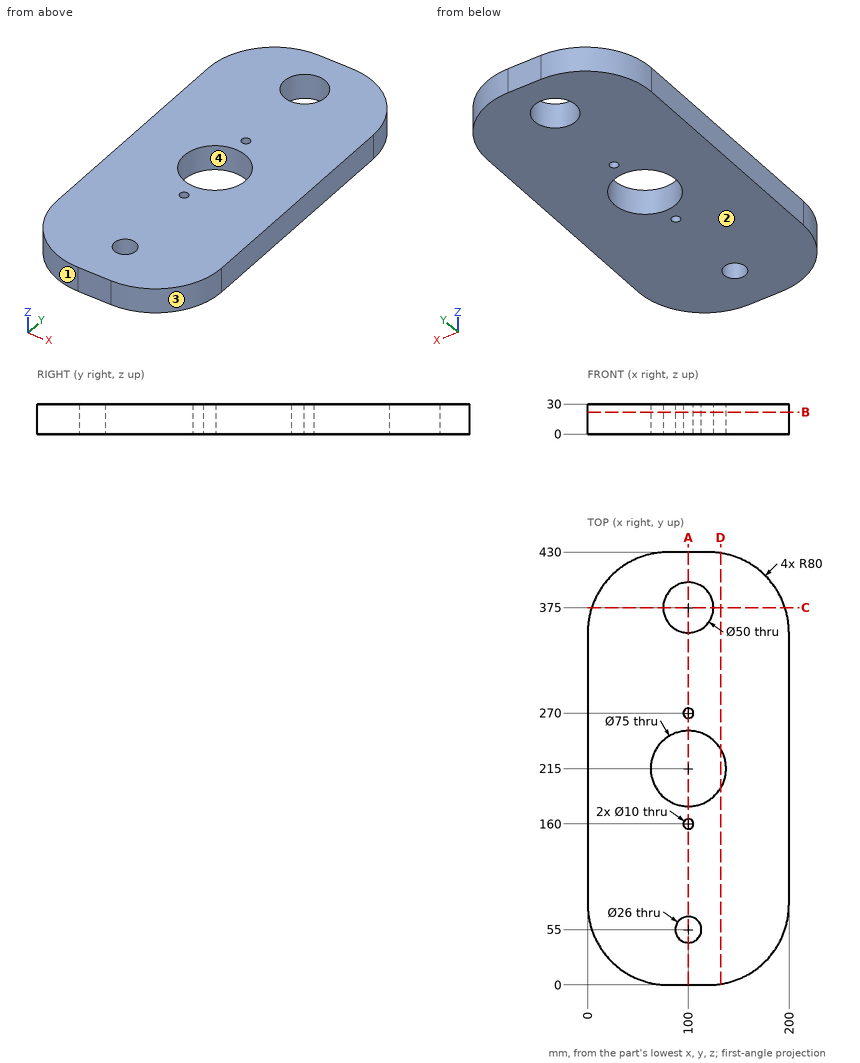
Here's the drawing with two shaded views (mm, measured from the low corner). I have some questions. Give positions to 0.01 mm unless a question says otherwise; leave off trailing zeros. Order: outer loops, then holes, each group sorted by start corner. A loop starts at its lowest first (then second) coordinate and runs counter-clockwise, first axis right, second up.
Q1. We'd pull the mould along X, two halves only. Please class the marked faces 1, 2, 3 and 4: +X half, -X half, draft (parallel to the pull), parting line (faces both ways), or undercut.
Q2. Suppose I cut it at A-A, the plane x = 100. Write out the boundary of the cut face in (y, z).
Q3. Suppose I cut it at D-D, the plane x = 132. Write out the boundary of the cut face in (y, z), and give its area (3 significant figures).
Q4. Suppose I cut it at C-C, the plane y = 375. Write out the boundary of the cut face in (x, z), and give its area (3 significant figures).
Q5. Suppose I cut it at B-B, the plane z = 22. Write out the boundary of the cut face in (x, y), and give its area (3 significant figures).
Q6. If I drill on line 1 along Y through (x, z) = (100, 19.5); line 2 along X through (y, z) = (270, 23); line 3 along Y through (x, z) = (104.5, 17.25), over which ranges is the centre line in solid material (lowest first)?
Q7. I'm going to push flat-ended pins straight in: P1, Ø8, axis at x = 41, z = 11, coming from the +Y side; P2, Ø5, axis at x = 32, z = 25, coming from the +Y side; P3, Ø5, axis at x = 143.5, z = 12.5, coming from the -Y side. Where does each tip first touch, or does it pass through?
Solution:
1. face 1: -X half
1. face 2: draft
1. face 3: +X half
1. face 4: undercut
2. outline: (0, 0) - (42, 0) - (42, 30) - (0, 30) - close; (68, 0) - (155, 0) - (155, 30) - (68, 30) - close; (165, 0) - (177.5, 0) - (177.5, 30) - (165, 30) - close; (252.5, 0) - (265, 0) - (265, 30) - (252.5, 30) - close; (275, 0) - (350, 0) - (350, 30) - (275, 30) - close; (400, 0) - (430, 0) - (430, 30) - (400, 30) - close
3. outline: (0.91, 0) - (195.45, 0) - (195.45, 30) - (0.91, 30) - close; (234.55, 0) - (429.09, 0) - (429.09, 30) - (234.55, 30) - close
3. area: 11,700 mm2
4. outline: (4.01, 0) - (75, 0) - (75, 30) - (4.01, 30) - close; (125, 0) - (195.99, 0) - (195.99, 30) - (125, 30) - close
4. area: 4,260 mm2
5. outline: (0, 80) arc R80 ccw to (80, 0) - (120, 0) arc R80 ccw to (200, 80) - (200, 350) arc R80 ccw to (120, 430) - (80, 430) arc R80 ccw to (0, 350) - close; hole circle Ø75 at (100, 215); hole circle Ø50 at (100, 375); hole circle Ø26 at (100, 55); hole circle Ø10 at (100, 160); hole circle Ø10 at (100, 270)
5. area: 73,400 mm2
6. line 1: y = 0 to 42, 68 to 155, 165 to 177.5, 252.5 to 265, 275 to 350, 400 to 430
6. line 2: x = 0 to 95, 105 to 200
6. line 3: y = 0 to 42.8, 67.2 to 157.82, 162.18 to 177.77, 252.23 to 267.82, 272.18 to 350.41, 399.59 to 430
7. P1: stops at y = 421.94
7. P2: stops at y = 415.8
7. P3: stops at y = 2.81
